Work out the finished part from the listing and answer in its coordinate system (mm). A direction names the side the tool comes from. Give positions to 0.01 mm unless a question says otherwise; leave off trailing zeros. Loops run counter-clockwise (first coordinate to the right, second up) from the corner with the lowest first, then second, coordinate; pieces in that order, holes last. Notation, with made-up numbers: (27.25, 46) - (45.25, 46) arc R24 ccw to (45.25, 83) - close; hole circle Ø10 at (36.25, 21.25). An arc over 180 degrees is marked (long way). One line per question, with ' | ' between items.
from build123d import *

# Parameters (mm, degrees)
SKETCH1_R           = 75
BOSS_EXTRUDE1_DEPTH = 40
SKETCH3_W           = 75
SKETCH3_H           = 75
BOSS_EXTRUDE2_DEPTH = 347.5
CUT_EXTRUDE1_DEPTH  = 80
SKETCH4_R           = 22.5
CUT_EXTRUDE2_DEPTH  = 80
CUT_EXTRUDE3_DEPTH  = 80


with BuildPart() as part:
    # Sketch1 → Boss-Extrude1 (new body)
    with BuildSketch(Plane(origin=(0, 0, 0), x_dir=(1, 0, 0), z_dir=(0, 1, 0))):
        with Locations(Location((0, 0, 0), (0, 0, 270))):
            Circle(SKETCH1_R)
    extrude(amount=BOSS_EXTRUDE1_DEPTH)

    # Sketch3 → Boss-Extrude2 (add)
    with BuildSketch(Plane(origin=(0, 40, 0), x_dir=(1, 0, 0), z_dir=(0, 1, 0))):
        Rectangle(SKETCH3_W, SKETCH3_H)
    extrude(amount=BOSS_EXTRUDE2_DEPTH)

    # Sketch5 → Cut-Extrude1 (cut)
    with BuildSketch(Plane.ZY.offset(37.5)):
        with BuildLine():
            Line((37.5, 387.5), (0, 387.5))
            ThreePointArc((0, 387.5), (26.516504294, 376.516504294), (37.5, 350))
            Line((37.5, 350), (37.5, 387.5))
        make_face()
        with BuildLine():
            Line((-37.5, 387.5), (-37.5, 350))
            ThreePointArc((-37.5, 350), (-26.516504294, 376.516504294), (0, 387.5))
            Line((0, 387.5), (-37.5, 387.5))
        make_face()
    extrude(amount=-CUT_EXTRUDE1_DEPTH, mode=Mode.SUBTRACT)

    # Sketch4 → Cut-Extrude2 (cut)
    with BuildSketch(Plane.ZY.offset(37.5)):
        with Locations((0, 350)):
            Circle(SKETCH4_R)
    extrude(amount=-CUT_EXTRUDE2_DEPTH, mode=Mode.SUBTRACT)

    # Sketch6 → Cut-Extrude3 (cut)
    with BuildSketch(Plane.XY.offset(37.5)):
        with BuildLine():
            Line((27.5, 401.577624338), (-27.5, 401.577624338))
            Line((-27.5, 401.577624338), (-27.5, 106.661183131))
            ThreePointArc((-27.5, 106.661183131), (0, 79.161183131), (27.5, 106.661183131))
            Line((27.5, 106.661183131), (27.5, 401.577624338))
        make_face()
    extrude(amount=-CUT_EXTRUDE3_DEPTH, mode=Mode.SUBTRACT)


solid = part.part
1. Find section C-C on z = -42. Write down the section's boundary in (x, y), then the cut area to 3 significant figures.
Evaluation:
outline: (-62.14, 0) - (62.14, 0) - (62.14, 40) - (-62.14, 40) - close | area: 4,970 mm2
2. Determine the mould class of faces 1 (the cylindrical face through (-0.605, 79.168, 0.525)), 2 (the cylindrical face through (32.43, 372.31, -2.93)), 3 (the flat face through (-28, 160, -37.5)) for opening direction Z: +Z half, -Z half, draft (parallel to the pull), parting line (faces both ways), or undercut.
Evaluation:
face 1: draft | face 2: undercut | face 3: -Z half
3. Find section A-A on y = 119. Write down the section's boundary in (x, z).
Evaluation:
outline: (-37.5, -37.5) - (-27.5, -37.5) - (-27.5, 37.5) - (-37.5, 37.5) - close; (27.5, -37.5) - (37.5, -37.5) - (37.5, 37.5) - (27.5, 37.5) - close
4. Which of the six approach directions +Z, -Z, +X, -X, +Y, -Y give full straight-line access (tool end or side, diameter ignored) to faces 4 (the flat face through (37.5, 211, 1)), 5 (the flat face through (27.5, 245, 1)), 6 (the flat face through (-37.5, 211, 1)), 7 (the flat face through (-28, 160, 37.5)), 8 (the flat face through (-49, 40, -1))?
Evaluation:
face 4: +Z, -Z, +X, +Y | face 5: +Z, -Z, +Y | face 6: +Z, -Z, -X, +Y | face 7: +Z, +X, -X, +Y | face 8: +Y
5. Find section B-B on x = 0. Write down the section's boundary in (y, z), then the cut area to 3 significant figures.
Evaluation:
outline: (0, -75) - (40, -75) - (40, -37.5) - (79.16, -37.5) - (79.16, 37.5) - (40, 37.5) - (40, 75) - (0, 75) - close | area: 8,940 mm2
6. Consider L1, parallel to X at y = 276.5, z = 19; L2, parallel to Y at x = -63, z = 36.5; L3, parallel to Y at x = 29, z = 20. Determine where each line is inside the solid, lowest interval first.
Evaluation:
L1: -37.5 to -27.5, 27.5 to 37.5 | L2: 0 to 40 | L3: 0 to 339.69, 360.31 to 381.72
7. Find section D-D on x = -44.5. Write down the section's boundary in (y, z).
Evaluation:
outline: (0, -60.37) - (40, -60.37) - (40, 60.37) - (0, 60.37) - close
8. Flat-ended cylindrical pins translate along their axes: pin 1 (22.5 mm diameter, centred on x = -18, y = 204.5, fed in from +Z); pin 2 (2 mm diameter, centred on y = 313.5, z = 35.5, fed in from +X); pin 3 (5 mm diameter, centred on x = 5, z = -5.5, fed in from +Y); pin 4 (22.5 mm diameter, centred on x = 9.5, y = 182, fed in from -Z). Find the tip coordinate at first contact, or state that the pin passes through.
Evaluation:
pin 1: z = 37.5 | pin 2: x = 37.5 | pin 3: y = 80.2 | pin 4: through
